from build123d import *

# Parameters (mm, degrees)
SKETCH1_W                = 6
SKETCH1_H                = 1.2
SKETCH1_W_2              = 1.2
SKETCH1_H_2              = 4.3
REVOLVE1_ANGLE           = 180
REVOLVE2_START           = 4.3
REVOLVE2_DEPTH           = 2.7
SKETCH3_W                = 6.5
SKETCH3_H                = 1.5
CUT_EXTRUDE1_DEPTH       = 10
CUT_EXTRUDE2_DEPTH       = 10
SKETCH7_W                = 2.9
SKETCH7_H                = 1.2
BOSS_EXTRUDE3_DEPTH      = 5
BOSS_EXTRUDE4_DEPTH      = 0.6
FILLET1_R                = 0.5
SKETCH9_W                = 3.4
SKETCH9_H                = 5.5
SKETCH9_W_2              = 1.2
SKETCH9_H_2              = 3
BOSS_EXTRUDE5_DEPTH      = 2.6
SKETCH11_W               = 1.2
SKETCH11_H               = 3
CUT_EXTRUDE3_DEPTH       = 3.6
CHAMFER2_SIZE            = 0.5
CHAMFER3_SIZE            = 0.5
CHAMFER2_OF_MIRROR2_SIZE = 0.5
CHAMFER3_OF_MIRROR2_SIZE = 0.5
SKETCH5_W                = 2
SKETCH5_H                = 2
CUT_EXTRUDE4_DEPTH       = 3.6


# Read off the part's stored shape, not the designer's step: Revolve2
with BuildPart() as part:
    # Sketch1 → Revolve1 (revolve)
    with BuildSketch(Plane.XY):
        with Locations((3, -0.6)):
            Rectangle(SKETCH1_W, SKETCH1_H)
        with Locations((6.6, -0.6)):
            Rectangle(SKETCH1_W_2, SKETCH1_H)
        with Locations((6.6, 2.15)):
            Rectangle(SKETCH1_W_2, SKETCH1_H_2)
    revolve(axis=Axis((0, -1.2, 0), (0, 1, 0)), revolution_arc=REVOLVE1_ANGLE)

    # Revolve2 outline → Revolve2 (add)
    with BuildSketch(Plane(origin=(0, 0, 0), x_dir=(1, 0, 0), z_dir=(0, 1, 0)).offset(REVOLVE2_START)):
        with BuildLine():
            ThreePointArc((3.7, 6.176568627), (0, 7.2), (-3.7, 6.176568627))
            Line((-3.7, 6.176568627), (-3.7, 4.723346271))
            ThreePointArc((-3.7, 4.723346271), (0, 6), (3.7, 4.723346271))
            Line((3.7, 4.723346271), (3.7, 6.176568627))
        make_face()
    extrude(amount=REVOLVE2_DEPTH)

    # Sketch3 → Cut-Extrude1 (cut)
    with BuildSketch(Plane.XY):
        with Locations((0, 0.75)):
            Rectangle(SKETCH3_W, SKETCH3_H)
    extrude(amount=-CUT_EXTRUDE1_DEPTH, mode=Mode.SUBTRACT)

    # Sketch4 → Cut-Extrude2 (cut)
    with BuildSketch(Plane(origin=(0, 0, 0), x_dir=(1, 0, 0), z_dir=(0, 1, 0))):
        Polygon((-1.45, 3.3), (-3.6, 3.3), (-3.6, 0), (3.6, 0), (3.6, 3.3), (1.45, 3.3), (1.45, 0.8), (-1.45, 0.8), align=None)
    extrude(amount=-CUT_EXTRUDE2_DEPTH, mode=Mode.SUBTRACT)

    # Sketch7 → Boss-Extrude3 (add)
    with BuildSketch(Plane.XZ.offset(1.2)):
        with Locations((0, -1.4)):
            Rectangle(SKETCH7_W, SKETCH7_H)
    extrude(amount=BOSS_EXTRUDE3_DEPTH)

    # Sketch8 → Boss-Extrude4 (add, symmetric)
    with BuildSketch(Plane(origin=(0, 0, 0), x_dir=(0, 0, -1), z_dir=(1, 0, 0))):
        Polygon((2, -6.2), (6, -1.2), (2, -1.2), align=None)
    extrude(amount=BOSS_EXTRUDE4_DEPTH, both=True)

    # Fillet1
    fillet1_edges = [part.edges().sort_by_distance(p)[0] for p in [
        (-1.45, -6.2, -1.4),
        (1.45, -6.2, -1.4),
    ]]
    fillet(fillet1_edges, radius=FILLET1_R)

    # Sketch9 → Boss-Extrude5 (add)
    with BuildSketch(Plane(origin=(6, 0, 0), x_dir=(0, 0, -1), z_dir=(1, 0, 0))):
        with Locations((0.8, 1.55)):
            Rectangle(SKETCH9_W, SKETCH9_H)
        with Locations((0.6, 1.55)):
            Rectangle(SKETCH9_W_2, SKETCH9_H_2, mode=Mode.SUBTRACT)
    boss_extrude5 = extrude(amount=BOSS_EXTRUDE5_DEPTH)

    # Sketch11 → Cut-Extrude3 (cut)
    with BuildSketch(Plane(origin=(8.6, 0, 0), x_dir=(0, 0, -1), z_dir=(1, 0, 0))):
        with Locations((0.6, 1.55)):
            Rectangle(SKETCH11_W, SKETCH11_H)
    cut_extrude3 = extrude(amount=-CUT_EXTRUDE3_DEPTH, mode=Mode.SUBTRACT)

    # Chamfer2
    chamfer2_edges = [part.edges().sort_by_distance(p)[0] for p in [
        (8.6, 1.55, 0.9),
    ]]
    chamfer(chamfer2_edges, length=CHAMFER2_SIZE)

    # Chamfer3
    chamfer3_edges = [part.edges().sort_by_distance(p)[0] for p in [
        (8.6, 1.55, -2.5),
    ]]
    chamfer(chamfer3_edges, length=CHAMFER3_SIZE)

    # Mirror2: Boss-Extrude5, Cut-Extrude3 across plane
    add(boss_extrude5.mirror(Plane(origin=(0, 0, 0), x_dir=(0, 0, 1), z_dir=(1, 0, 0))))
    add(cut_extrude3.mirror(Plane(origin=(0, 0, 0), x_dir=(0, 0, 1), z_dir=(1, 0, 0))), mode=Mode.SUBTRACT)

    # Chamfer2 of Mirror2
    chamfer2_of_mirror2_edges = [part.edges().sort_by_distance(p)[0] for p in [
        (-8.6, 1.55, 0.9),
    ]]
    chamfer(chamfer2_of_mirror2_edges, length=CHAMFER2_OF_MIRROR2_SIZE)

    # Chamfer3 of Mirror2
    chamfer3_of_mirror2_edges = [part.edges().sort_by_distance(p)[0] for p in [
        (-8.6, 1.55, -2.5),
    ]]
    chamfer(chamfer3_of_mirror2_edges, length=CHAMFER3_OF_MIRROR2_SIZE)

    # Sketch5 → Cut-Extrude4 (cut)
    with BuildSketch(Plane(origin=(0, 0, 0), x_dir=(1, 0, 0), z_dir=(0, 1, 0))):
        with Locations((4.6, 1)):
            Rectangle(SKETCH5_W, SKETCH5_H)
        with Locations((-4.6, 1)):
            Rectangle(SKETCH5_W, SKETCH5_H)
    extrude(amount=-CUT_EXTRUDE4_DEPTH, mode=Mode.SUBTRACT)


solid = part.part
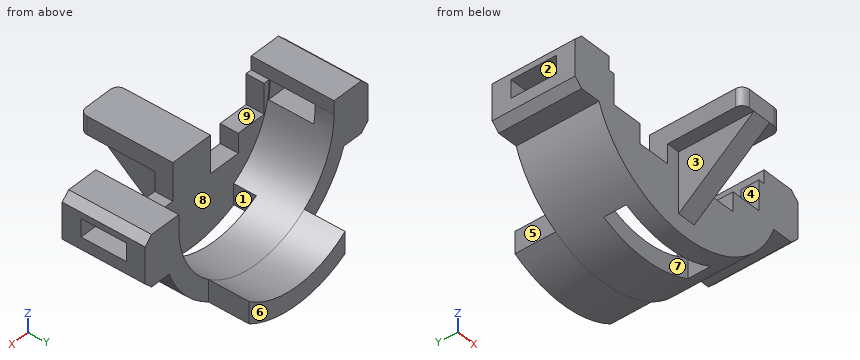
Check sheet for the modelled part. Datum: model origin and axes. Units: mm. Face numbers are marked on the shaded views. A direction names the side the tool comes from. Give positions to 0.01 mm unless a question says otherwise; leave off trailing zeros. Order: outer loops, then holes, each group sorted by start corner. A loop starts at its lowest first (then second) coordinate and runs counter-clockwise, first axis right, second up. Notation, with made-up numbers: (37.25, -33.5) - (72.25, -33.5) arc R25 ccw to (72.25, 5.5) - close; hole circle Ø6 at (-30, 15.25). An arc over 180 degrees is marked (long way). Answer as CSV lines item,"result".
1. Section check A-A (x = 0). Record the boundary of the cut face in (y, z).
Result sheet:
outline,"(-6.2, -2) - (-1.2, -6) - (-1.2, -7.2) - (0, -7.2) - (0, -0.8) - (-6.2, -0.8) - close; (1.5, -7.2) - (7, -7.2) - (7, -6) - (1.5, -6) - close"
2. Section check B-B (y = -3.5). Record the boundary of the cut face in (x, z), then the cut area to 3 significant figures.
Result sheet:
outline,"(-1.45, -2) - (-0.6, -2) - (-0.6, -4.16) - (0.6, -4.16) - (0.6, -2) - (1.45, -2) - (1.45, -0.8) - (-1.45, -0.8) - close"
area,"6.07 mm²"
3. Section check D-D (x = -6.5). Record the boundary of the cut face in (y, z), then the cut area to 3 significant figures.
Result sheet:
outline,"(-1.2, -3.1) - (4.3, -3.1) - (4.3, 0.9) - (-1.2, 0.9) - close; hole (0.05, -1.2) - (3.05, -1.2) - (3.05, 0) - (0.05, 0) - close"
area,"18.4 mm²"
4. Scan lines: probe 1 along X at (y, z) = (-0.75, 0.25); probe 2 along X at (y, z) = (-1, -0.5); probe 3 along X at (y, z) = (-2, -3.25). Record each from-to range of solid material in increasing order. Write a range as from..to.
Result sheet:
probe 1,"-8.6..-6, 6..8.6"
probe 2,"-8.6..-5.6, 5.6..8.6"
probe 3,"-0.6..0.6"
5. Mould release check, pull along Y, two halves, no side actions. Record for the marked faces 6, 7, 8 and 9: released by +Y, released by -Y, zero draft, split by the parting line, or undercut.
Result sheet:
face 6,"released by +Y"
face 7,"undercut"
face 8,"undercut"
face 9,"zero draft"
6. Tool access check on the marked faces 1, 2, 3, 4 and 5. Record the directions out of +Z, -Z, +X, -X, +Y, -Y that give a thin tool (end or side, any length) a straight path to the whole face; none if there is none.
Result sheet:
face 1,"+Z, -Z"
face 2,"+X, -X"
face 3,"-Z, -X, -Y"
face 4,"+Z, +Y, -Y"
face 5,"+Z, -Z, -X, +Y"
7. Section check C-C (z = -5.75). Record the boundary of the cut face in (x, y).
Result sheet:
outline,"(-4.33, -1.2) - (-0.6, -1.2) - (-0.6, -1.51) - (0.6, -1.51) - (0.6, -1.2) - (4.33, -1.2) - (4.33, 4.3) - (3.7, 4.3) - (3.7, 7) - (1.71, 7) - (1.71, 1.5) - (3.25, 1.5) - (3.25, 0) - (-3.25, 0) - (-3.25, 1.5) - (-1.71, 1.5) - (-1.71, 7) - (-3.7, 7) - (-3.7, 4.3) - (-4.33, 4.3) - close"
8. Go/stop test with flat-tipped pins: P1, Ø2, axis at x = 3.5, y = -1.5, coming from the -Z side; P2, Ø4.5, axis at y = -3.5, z = -4.5, coming from the -X side; P3, Ø1.3, axis at x = -4.5, y = -0.5, coming from the +Z side. Record where each tip stops, or that it passes through.
Result sheet:
P1,"z = -6.73"
P2,"x = -0.6"
P3,"z = -2"
